```python
from build123d import *

# Parameters (mm, degrees)
SKETCH2_W                     = 200
SKETCH2_H                     = 84
BOSS_EXTRUDE1_DEPTH           = 5
SKETCH5_W                     = 13.375130616
SKETCH5_H                     = 29
BOSS_EXTRUDE2_DEPTH           = 5
CBORE_FOR_M5_SHCS4_AT_2_COUNT = 2
CBORE_FOR_M5_SHCS4_AT_2_PITCH = 15
CHAMFER1_SIZE                 = 5


with BuildPart() as part:
    # Sketch2 → Boss-Extrude1 (new body)
    with BuildSketch(Plane(origin=(0, 0, 0), x_dir=(1, 0, 0), z_dir=(0, 1, 0))):
        Rectangle(SKETCH2_W, SKETCH2_H)
    extrude(amount=BOSS_EXTRUDE1_DEPTH)

    # Sketch5 → Boss-Extrude2 (add)
    with BuildSketch(Plane(origin=(0, 5, 0), x_dir=(1, 0, 0), z_dir=(0, 1, 0))):
        with Locations((0, 27.5)):
            Rectangle(SKETCH5_W, SKETCH5_H)
    extrude(amount=BOSS_EXTRUDE2_DEPTH)

    # Sketch4 → CBORE for M5 SHCS4 (revolve, cut)
    with BuildSketch(Plane(origin=(0, 0, -20), x_dir=(0, 0, -1), z_dir=(1, 0, 0))):
        Polygon((0, 0), (0, 10), (2.9, 10), (2.9, 5), (5, 5), (5, 0.020977491), (5.025, 0), align=None)
    cbore_for_m5_shcs4 = revolve(axis=Axis((0, -6.35, -20), (0, 1, 0)), mode=Mode.SUBTRACT)

    # CBORE for M5 SHCS4 at 2: CBORE for M5 SHCS4 ×2
    with Locations(*[(0, 0, -i * CBORE_FOR_M5_SHCS4_AT_2_PITCH) for i in range(1, CBORE_FOR_M5_SHCS4_AT_2_COUNT)]):
        add(cbore_for_m5_shcs4, mode=Mode.SUBTRACT)

    # Chamfer1
    chamfer1_edges = [part.edges().sort_by_distance(p)[0] for p in [
        (-6.687565308, 5, -27.5),
        (0, 5, -13),
        (6.687565308, 5, -27.5),
    ]]
    chamfer(chamfer1_edges, length=CHAMFER1_SIZE - 0.0001)  # a hair under: the kernel refuses the full size


solid = part.part
```
Input: part model. Units: mm. Frame: model coordinates. A direction names the side the tool comes from. Round coordinates to 2 decimals unless told otherwise and drop trailing zeros. Order: outer loops, then holes, each group sorted by start corner. A loop starts at its lowest first (then second) coordinate and runs counter-clockwise, first axis right, second up. Notation, with made-up numbers: (64, 76.25) - (103, 76.25) arc R29 ccw to (103, 98.25) - close; hole circle Ø8 at (78.5, 67). An arc over 180 degrees is marked (long way). Answer in a Markdown table with one row per item.
Item 1: Pin query (flat end, axial travel): pin 1 (4 mm diameter, centred on y = 8, z = 17, fed in from -X); pin 2 (6.5 mm diameter, centred on x = 0, z = -20, fed in from -Y); pin 3 (1 mm diameter, centred on x = -74, z = -10, fed in from +Y). Return the tip coordinate at first contact, or that it passes through.
Model answer:
| item | result |
|---|---|
| pin 1 | passes through |
| pin 2 | stops at y = 5 |
| pin 3 | stops at y = 5 |
Item 2: Mould query, pull axis X, two halves, no side actions, for faces 1 (the flat face through (-1, 2, 42)), 2 (the flat face through (-100, 2, 1)), 3 (the cylindrical face through (0, 2, -30)), 4 (the flat face through (100, 2, 1)). Classes: released by +X, released by -X, zero draft, split by the parting line, or undercut.
Model answer:
| item | result |
|---|---|
| face 1 | zero draft |
| face 2 | released by -X |
| face 3 | undercut |
| face 4 | released by +X |
Item 3: Reachability of faces 5 (the cylindrical face through (-0.1, 7.5, -17.1)), 6 (the cylindrical face through (0, 2, -15)) from +Z, -Z, +X, -X, +Y, -Y: full face, straight path, thin tool, end or side. Return the list, or none.
Model answer:
| item | result |
|---|---|
| face 5 | +Y, -Y |
| face 6 | -Y |
Item 4: Line query: line 1 (Z direction, x = 0, y = 2.15); line 2 (Z direction, x = 0, y = 9); line 3 (X direction, y = 1.4, z = -35). Output: solid intervals per line, ascending.
Model answer:
| item | result |
|---|---|
| line 1 | z = -42 to -40, -30 to -25, -15 to 42 |
| line 2 | z = -42 to -37.9, -32.1 to -22.9, -17.1 to -12 |
| line 3 | x = -100 to -5, 5 to 100 |
Item 5: Section query C-C (y = 6.75). Return the cut outline in (x, z).
Model answer:
| item | result |
|---|---|
| outline | (-9.94, -42) - (9.94, -42) - (9.94, -9.75) - (-9.94, -9.75) - close; hole circle Ø5.8 at (0, -35); hole circle Ø5.8 at (0, -20) |
Item 6: Section query A-A (x = 0). Give the number of separate pieces and of enclosed holes in the cut face, then the cut area to 3 significant figures.
Model answer:
| item | result |
|---|---|
| separate pieces | 3 |
| enclosed holes | 0 |
| area | 419 mm² |
Item 7: Section query D-D (z = -2). Return the cut outline in (x, y).
Model answer:
| item | result |
|---|---|
| outline | (-100, 0) - (100, 0) - (100, 5) - (-100, 5) - close |
